```python
from build123d import *

# Parameters (mm, degrees)
SKETCH_1_R          = 7
EXTRUDE_1_DEPTH     = 6
SKETCH_2_R          = 2.5
CUT_EXTRUDE_1_DEPTH = 12.575836903
FILLET_1_R          = 0.2


with BuildPart() as part:
    # 草图1 → 凸台-拉伸1 (new body)
    with BuildSketch(Plane.XY):
        Circle(SKETCH_1_R)
    extrude(amount=EXTRUDE_1_DEPTH)

    # 草图2 → 切除-拉伸1 (cut, through all)
    with BuildSketch(Plane.XY.offset(6)):
        Circle(SKETCH_2_R)
    extrude(amount=-CUT_EXTRUDE_1_DEPTH, mode=Mode.SUBTRACT)

    # 圆角1
    fillet_1_edges = [part.edges().sort_by_distance(p)[0] for p in [
        (-7, 0, 0),
        (-7, 0, 6),
        (-2.5, 0, 0),
        (-2.5, 0, 6),
    ]]
    fillet(fillet_1_edges, radius=FILLET_1_R)


solid = part.part
```
Verification items for the finished model (mm, model axes). Coordinates: 2 decimals unless noted, no trailing zeros. Loops run counter-clockwise (first coordinate to the right, second up) from the corner with the lowest first, then second, coordinate; pieces in that order, holes last. Notation, with made-up numbers: (75.5, -27.5) - (90.5, -27.5) arc R18 ccw to (90.5, 1.5) - close; hole circle Ø7 at (2, 28). An arc over 180 degrees is marked (long way). Return JSON: item names as keys, results as strings.
1. Go/stop test with flat-tipped pins: pin 1 (3 mm diameter, centred on x = 0, y = 0, fed in from -Z); pin 2 (1 mm diameter, centred on y = 3.5, z = 3, fed in from -X); pin 3 (1.5 mm diameter, centred on y = -4, z = 4.5, fed in from +X). Record where each tip stops, or that it passes through.
Established:
{"pin 1": "passes through", "pin 2": "stops at x = -6.32", "pin 3": "stops at x = 6.2"}
2. Section check A-A, the plane x = 0. Record the boundary of the cut face in (y, z).
Established:
{"outline": "(-7, 0.2) arc R0.2 ccw to (-6.8, 0) - (-2.7, 0) arc R0.2 ccw to (-2.5, 0.2) - (-2.5, 5.8) arc R0.2 ccw to (-2.7, 6) - (-6.8, 6) arc R0.2 ccw to (-7, 5.8) - close; (2.5, 0.2) arc R0.2 ccw to (2.7, 0) - (6.8, 0) arc R0.2 ccw to (7, 0.2) - (7, 5.8) arc R0.2 ccw to (6.8, 6) - (2.7, 6) arc R0.2 ccw to (2.5, 5.8) - close"}
3. Thickness scan on L1, parallel to Y at x = 0, z = 2.15; L2, parallel to X at y = 0.5, z = 1.25. Record the ranges inside material, lowest first.
Established:
{"L1": "y = -7 to -2.5, 2.5 to 7", "L2": "x = -6.98 to -2.45, 2.45 to 6.98"}
4. Section check C-C, the plane z = 4.3. Record the boundary of the cut face in (x, y), then the cut area to 3 significant figures.
Established:
{"outline": "circle Ø14 at (0, 0); hole circle Ø5 at (0, 0)", "area": "134 mm2"}
